from build123d import *

# Parameters (mm, degrees)
BOSS_EXTRUDE1_DEPTH = 10
BOSS_EXTRUDE2_DEPTH = 20
SKETCH3_W           = 23.5
SKETCH3_H           = 12.5
CUT_EXTRUDE1_DEPTH  = 5
SKETCH4_R           = 1.25
CUT_EXTRUDE2_DEPTH  = 5
SKETCH5_R           = 2
CUT_EXTRUDE3_DEPTH  = 108.54650157


with BuildPart() as part:
    # Sketch1 → Boss-Extrude1 (new, symmetric)
    with BuildSketch(Plane.XY):
        Polygon((-24, 49.25), (0, 49.25), (0, -49.25), (-24, -49.25), (-24, -45.25), (-4, -45.25), (-4, 45.25), (-24, 45.25), align=None)
    extrude(amount=BOSS_EXTRUDE1_DEPTH, both=True)

    # Sketch2 → Boss-Extrude2 (add)
    with BuildSketch(Plane.XY.offset(10)):
        Polygon((0, -14), (38, -14), (38, -30), (0, -30), (0, -34), (42, -34), (42, -10), (0, -10), align=None)
    extrude(amount=-BOSS_EXTRUDE2_DEPTH)

    # Sketch3 → Cut-Extrude1 (cut)
    with BuildSketch(Plane(origin=(0, -10, 0), x_dir=(1, 0, 0), z_dir=(0, 1, 0))):
        with Locations((21, 0)):
            Rectangle(SKETCH3_W, SKETCH3_H)
    extrude(amount=-CUT_EXTRUDE1_DEPTH, mode=Mode.SUBTRACT)

    # Sketch4 → Cut-Extrude2 (cut)
    with BuildSketch(Plane(origin=(0, -10, 0), x_dir=(1, 0, 0), z_dir=(0, 1, 0))):
        with Locations(Location((35.5, 0, 0), (0, 0, 270))):
            Circle(SKETCH4_R)
        with Locations(Location((6.5, 0, 0), (0, 0, 270))):
            Circle(SKETCH4_R)
    extrude(amount=-CUT_EXTRUDE2_DEPTH, mode=Mode.SUBTRACT)

    # Sketch5 → Cut-Extrude3 (cut, through all)
    with BuildSketch(Plane(origin=(0, 49.25, 0), x_dir=(1, 0, 0), z_dir=(0, 1, 0))):
        with Locations(Location((-18, 5, 0), (0, 0, 180))):
            Circle(SKETCH5_R)
        with Locations(Location((-18, -5, 0), (0, 0, 180))):
            Circle(SKETCH5_R)
        with Locations(Location((-10, -5, 0), (0, 0, 180))):
            Circle(SKETCH5_R)
        with Locations(Location((-10, 5, 0), (0, 0, 180))):
            Circle(SKETCH5_R)
    extrude(amount=-CUT_EXTRUDE3_DEPTH, mode=Mode.SUBTRACT)


solid = part.part
The model under review builds one solid part; all positions refer to its coordinate system, in mm. A direction names the side the tool comes from. Give positions to 0.01 mm unless a question says otherwise; leave off trailing zeros. Order: outer loops, then holes, each group sorted by start corner. A loop starts at its lowest first (then second) coordinate and runs counter-clockwise, first axis right, second up. Notation, with made-up numbers: (31, 87.25) -> (81, 87.25) arc R10 ccw to (81, 91.25) -> close; hole circle Ø11 at (-6, -20). An arc over 180 degrees is marked (long way). Write item = value, one per line. Start each with the question number.
(1) For pin 1 Ø2 at (x, z) = (35.5, 0) entering from -Y; pin 2 Ø1 at (x, z) = (16.5, -5.5) entering from +Y; pin 3 Ø6 at (y, z) = (-21.5, 3.5) entering from -X, all flat-tipped, find the tip position at first contact; note any pin that passes through.
(2) Take a section at A-A (x = -18). Write out the cut boundary in (y, z).
(3) For L1, parallel to Z at x = -18, y = -46.7; L2, parallel to Y at x = 35, z = -1.5; L3, parallel to Y at x = -8.5, z = -9, list the stretches that pass through material, from the lowest coordinate up. Write a range as from..to.
(4) Draft analysis for pull direction X (two halves, no side actions). For faces 6 (the flat face through (42, -22, 0)), 7 (the flat face through (-4, -1, 0)), 8 (the flat face through (0, -22, 0)), state which applies: +X half, -X half, draft (parallel to the pull), parting line (faces both ways), or undercut.
(5) Take a section at C-C (z = 0). Write out the cut boundary in (x, y), plus the area to 3 significant figures.
(6) Tool access review of faces 1 (the flat face through (19, -14, 7)), 2 (the flat face through (-14, -45.25, 0)), 3 (the flat face through (21, -12, 6.25)), 4 (the flat face through (0, 20, 0)), 5 (the cylindrical face through (-16, -47, 5)): name each direction out of +Z, -Z, +X, -X, +Y, -Y from which nothing blocks a thin tool from reaching the whole face with its end or side.
(7) Take a section at B-B (y = -24). Write out the cut boundary in (x, z).
(8) Take a section at D-D (z = 8.5). Write out the cut boundary in (x, y), plus the area to 3 significant figures.
Returned:
q1.pin_1 = -34
q1.pin_2 = -30
q1.pin_3 = -4
q2.outline = (-49.25, -10) -> (-45.25, -10) -> (-45.25, -7) -> (-49.25, -7) -> close; (-49.25, -3) -> (-45.25, -3) -> (-45.25, 3) -> (-49.25, 3) -> close; (-49.25, 7) -> (-45.25, 7) -> (-45.25, 10) -> (-49.25, 10) -> close; (45.25, -10) -> (49.25, -10) -> (49.25, -7) -> (45.25, -7) -> close; (45.25, -3) -> (49.25, -3) -> (49.25, 3) -> (45.25, 3) -> close; (45.25, 7) -> (49.25, 7) -> (49.25, 10) -> (45.25, 10) -> close
q3.L1 = -10..-7, -3..3, 7..10
q3.L2 = -34..-30, -14..-10
q3.L3 = -49.25..-45.25, 45.25..49.25
q4.face_6 = +X half
q4.face_7 = -X half
q4.face_8 = undercut
q5.outline = (-24, -49.25) -> (0, -49.25) -> (0, -34) -> (42, -34) -> (42, -10) -> (36.75, -10) -> (36.75, -14) -> (38, -14) -> (38, -30) -> (0, -30) -> (0, -14) -> (5.25, -14) -> (5.25, -10) -> (0, -10) -> (0, 49.25) -> (-24, 49.25) -> (-24, 45.25) -> (-4, 45.25) -> (-4, -45.25) -> (-24, -45.25) -> close; (7.75, -14) -> (9.25, -14) -> (9.25, -10) -> (7.75, -10) -> close; (32.75, -14) -> (34.25, -14) -> (34.25, -10) -> (32.75, -10) -> close
q5.area = 840 mm²
q6.face_1 = +Z, -Z
q6.face_2 = +Z, -Z, -X
q6.face_3 = +Y
q6.face_4 = +Z, -Z, +X, +Y
q6.face_5 = +Y, -Y
q7.outline = (-4, -10) -> (0, -10) -> (0, 10) -> (-4, 10) -> close; (38, -10) -> (42, -10) -> (42, 10) -> (38, 10) -> close
q8.outline = (-24, -49.25) -> (0, -49.25) -> (0, -34) -> (42, -34) -> (42, -10) -> (0, -10) -> (0, 49.25) -> (-24, 49.25) -> (-24, 45.25) -> (-4, 45.25) -> (-4, -45.25) -> (-24, -45.25) -> close; hole (0, -30) -> (38, -30) -> (38, -14) -> (0, -14) -> close
q8.area = 954 mm²
